```python
from build123d import *

# Parameters (mm, degrees)
ESQUISSE2_W                 = 150
ESQUISSE2_H                 = 26
T_LE_DE_BASE_PLI_E1_DEPTH   = 4
PLI_START                   = -13
PLI_ESQUISS_1_DEPTH         = 26
PLI_ESQUISS_1_2_DEPTH       = 26
ESQUISSE9_R                 = 2.5
ESQUISSE9_R_2               = 1.25
BOSS_EXTRU_1_DEPTH          = 1.5
ENL_V_START                 = -4
ENL_V_MAT_EXTRU_1_OUTLINE_R = 1.25
ENL_V_MAT_EXTRU_1_DEPTH     = 4
ESQUISSE11_W                = 4
ESQUISSE11_H                = 26
BOSS_EXTRU_2_DEPTH          = 25
ESQUISSE12_R                = 2
ENL_V_MAT_EXTRU_5_DEPTH     = 148.599026321


# Read off the part's stored shape, not the designer's step: Pli esquissé1, Enlèv. mat.-Extru.1
# Sheet-metal steps are written as plain solids
with BuildPart() as part:
    # Esquisse2 → Tôle de base pliée1 (new body)
    with BuildSketch(Plane(origin=(0, 0, 0), x_dir=(1, 0, 0), z_dir=(0, 1, 0))):
        Rectangle(ESQUISSE2_W, ESQUISSE2_H)
    extrude(amount=-T_LE_DE_BASE_PLI_E1_DEPTH)

    # Pli esquissé1 outline → Pli esquissé1 (cut)
    with BuildSketch(Plane.XY.offset(PLI_START)):
        with BuildLine():
            Line((75, 0), (56.347473252, 0))
            Line((56.347473252, 0), (46.142385808, -3.714348068))
            ThreePointArc((46.142385808, -3.714348068), (45.344875155, -3.928040403), (44.522373197, -4))
            Line((44.522373197, -4), (75, -4))
            Line((75, -4), (75, 0))
        make_face()
    extrude(amount=PLI_ESQUISS_1_DEPTH, mode=Mode.SUBTRACT)

    # Pli esquiss_1 2 outline → Pli esquiss_1 2 (add)
    with BuildSketch(Plane.XY.offset(PLI_START)):
        with BuildLine():
            Line((56.347473252, 0), (73.884342049, 6.382898245))
            Line((73.884342049, 6.382898245), (72.516261476, 10.141668728))
            Line((72.516261476, 10.141668728), (44.774305234, 0.044422416))
            ThreePointArc((44.774305234, 0.044422416), (44.650282444, 0.011190609), (44.522373197, 0))
            Line((44.522373197, 0), (56.347473252, 0))
        make_face()
    extrude(amount=PLI_ESQUISS_1_2_DEPTH)

    # Esquisse9 → Boss.-Extru.1 (add)
    # profile 1 of 4: a face of its own
    with BuildSketch(Plane(origin=(5.223321668, -14.350958338, 0), x_dir=(0.9396926207859082, 0.34202014332566943, 0), z_dir=(-0.34202014332566943, 0.9396926207859082, 0))):
        with Locations(Location((55.111650787, 10.5, 0), (0, 0, 90))):
            Circle(ESQUISSE9_R)
        with Locations(Location((55.111650787, 10.5, 0), (0, 0, 180))):
            Circle(ESQUISSE9_R_2, mode=Mode.SUBTRACT)
    # profile 2 of 4: a face of its own
    with BuildSketch(Plane(origin=(5.223321668, -14.350958338, 0), x_dir=(0.9396926207859082, 0.34202014332566943, 0), z_dir=(-0.34202014332566943, 0.9396926207859082, 0))):
        with Locations(Location((68.611650787, 10.5, 0), (0, 0, 90))):
            Circle(ESQUISSE9_R)
        with Locations(Location((68.611650787, 10.5, 0), (0, 0, 180))):
            Circle(ESQUISSE9_R_2, mode=Mode.SUBTRACT)
    # profile 3 of 4: a face of its own
    with BuildSketch(Plane(origin=(5.223321668, -14.350958338, 0), x_dir=(0.9396926207859082, 0.34202014332566943, 0), z_dir=(-0.34202014332566943, 0.9396926207859082, 0))):
        with Locations((68.611650787, -10.5)):
            Circle(ESQUISSE9_R)
        with Locations((68.611650787, -10.5)):
            Circle(ESQUISSE9_R_2, mode=Mode.SUBTRACT)
    # profile 4 of 4: a face of its own
    with BuildSketch(Plane(origin=(5.223321668, -14.350958338, 0), x_dir=(0.9396926207859082, 0.34202014332566943, 0), z_dir=(-0.34202014332566943, 0.9396926207859082, 0))):
        with Locations((55.111650787, -10.5)):
            Circle(ESQUISSE9_R)
        with Locations((55.111650787, -10.5)):
            Circle(ESQUISSE9_R_2, mode=Mode.SUBTRACT)
    extrude(amount=BOSS_EXTRU_1_DEPTH)

    # Enlèv. mat.-Extru.1 outline → Enlèv. mat.-Extru.1 (cut)
    with BuildSketch(Plane(origin=(5.223321668, -14.350958338, 0), x_dir=(0.9396926207859082, 0.34202014332566943, 0), z_dir=(-0.34202014332566943, 0.9396926207859082, 0)).offset(ENL_V_START)):
        with Locations((68.611650787, 10.5)):
            Circle(ENL_V_MAT_EXTRU_1_OUTLINE_R)
        with Locations((68.611650787, -10.5)):
            Circle(ENL_V_MAT_EXTRU_1_OUTLINE_R)
        with Locations((55.111650787, 10.5)):
            Circle(ENL_V_MAT_EXTRU_1_OUTLINE_R)
        with Locations((55.111650787, -10.5)):
            Circle(ENL_V_MAT_EXTRU_1_OUTLINE_R)
    extrude(amount=ENL_V_MAT_EXTRU_1_DEPTH, mode=Mode.SUBTRACT)

    # Esquisse11 → Boss.-Extru.2 (add)
    with BuildSketch(Plane(origin=(0, 0, 0), x_dir=(1, 0, 0), z_dir=(0, 1, 0))):
        with Locations((-73, 0)):
            Rectangle(ESQUISSE11_W, ESQUISSE11_H)
    extrude(amount=BOSS_EXTRU_2_DEPTH)

    # Esquisse12 → Enlèv. mat.-Extru.5 (cut, through all)
    with BuildSketch(Plane(origin=(-71, 0, 0), x_dir=(0, 0, -1), z_dir=(1, 0, 0))):
        with Locations((-3, 7)):
            Circle(ESQUISSE12_R)
        with Locations((0, 17)):
            Circle(ESQUISSE12_R)
    extrude(amount=-ENL_V_MAT_EXTRU_5_DEPTH, mode=Mode.SUBTRACT)


solid = part.part
```
Can you work these out from the model? Positions are in its coordinate system, mm. A direction names the side the tool comes from. Give positions to 0.01 mm unless a question says otherwise; leave off trailing zeros. Loops run counter-clockwise (first coordinate to the right, second up) from the corner with the lowest first, then second, coordinate; pieces in that order, holes last. Notation, with made-up numbers: M -32,33 L 2,33 A15 ccw 2,54 Z; hole C -4,83.5 d6. An arc over 180 degrees is marked long. Use one line per item in the form item = value. Start each with the question number.
(1) I want a section at B-B, the plane z = 6.75. Write out the boundary of the cut face in (x, y).
(2) On a 3-axis mill with a long thin cutter (end or side, diameter ignored), from which of +Z, -Z, +X, -X, +Y, -Y can I reach the whole of each face in a straight line? I mean faces 1 (the flat face through (57.51, 6.276, 11.576)), 2 (the cylindrical face through (-73, 9, 3)), 3 (the cylindrical face through (70.215, 7.933, -11.747)). Say none if no direction works.
(3) Thinking about a two-plate mould opening in Y: for faces 4 (the flat face through (-11.9, -0.3, 13)), 5 (the cylindrical face through (68.964, 7.478, 10.445)), 6 (the cylindrical face through (67.1, 9, -10.2)), 7 (the flat face through (70.195, 10.893, -11.576)), which applies, released by +Y, released by -Y, zero draft, split by the parting line, or undercut?
(4) Please list where these lines run through material, in increasing order: line 1 (X direction, y = 12, z = 0.75); line 2 (Y direction, x = -22, z = 4.5); line 3 (Y direction, x = -72.85, z = 3).
(5) I'm going to push a flat-ended pin straight in: P1, Ø4, axis at x = -8, z = -3, coming from the +Y side. Where does the tip first touch, or does it pass through?
(6) I want a section at A-A, the plane y = 17. Write out the boundary of the cut face in (x, z), and give its area (3 significant figures).
Worked out:
q1.outline = M -75,-4 L 44.52,-4 A4.74 ccw 46.14,-3.71 L 73.88,6.38 L 72.52,10.14 L 44.77,0.04 A0.74 cw 44.52,0 L -71,0 L -71,25 L -75,25 Z
q2.face_1 = +Z, -Z, +Y
q2.face_2 = -X
q2.face_3 = none
q3.face_4 = zero draft
q3.face_5 = undercut
q3.face_6 = undercut
q3.face_7 = released by +Y
q4.line_1 = -75 to -71
q4.line_2 = -4 to 0
q4.line_3 = -4 to 5, 9 to 25
q5.P1 = 0
q6.outline = M -75,-13 L -71,-13 L -71,-2 L -75,-2 Z; M -75,2 L -71,2 L -71,13 L -75,13 Z
q6.area = 88.0 mm²
